Check sheet for the drawn part. Datum: minimum x, y, z corner. Units: mm. A direction names the side the tool comes from. Round coordinates to 2 decimals unless told otherwise and drop trailing zeros. Write each loop counter-clockwise with the first axis right and the second up, starting at its lowest first coordinate (ties: lowest second). Pieces come first, ordered by that corner, then holes. Notation, with made-up numbers: (-14, 46) - (-4, 46) arc R28 cw to (-4, 76) - close; hole circle Ø8 at (42, 63.25). An arc over 180 degrees is marked (long way). Write each question's results on one line, items separated by ' | '.
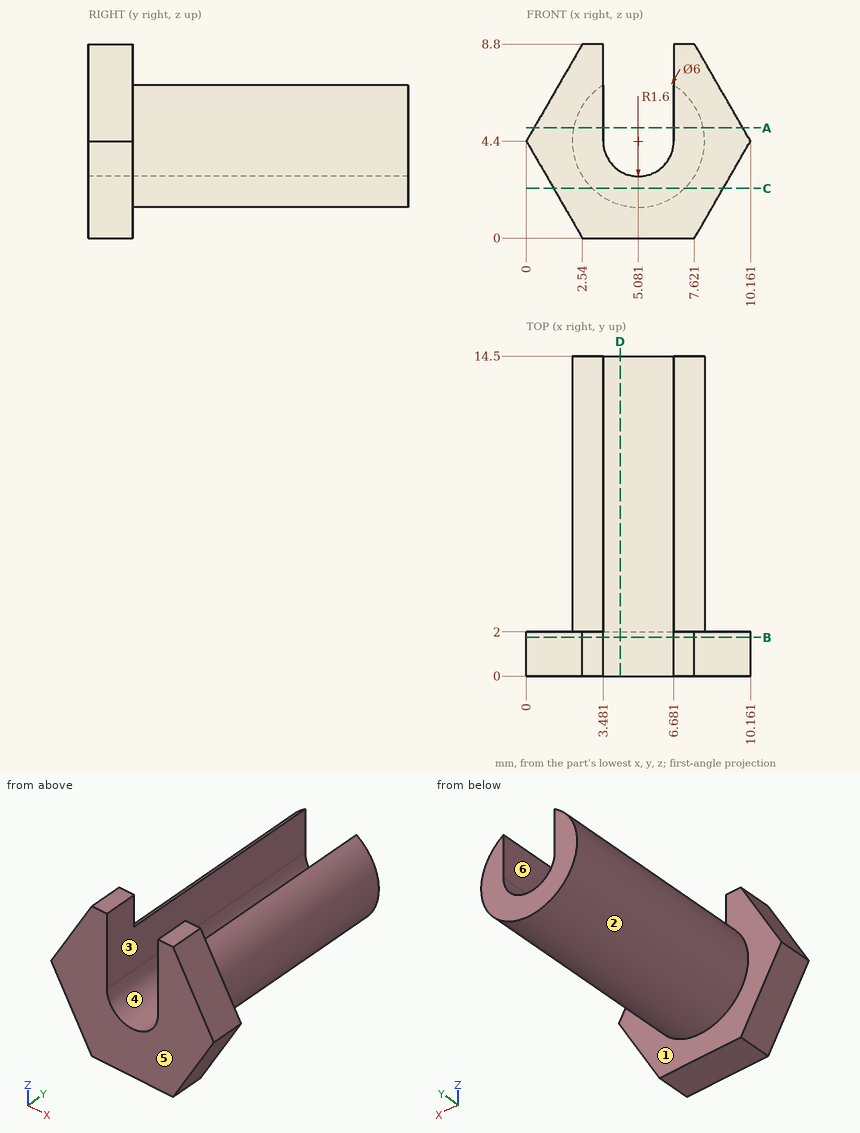
(1) Section check C-C (z = 2.25). Record the cut outline in (x, y).
Answer:
outline: (1.24, 0) - (8.92, 0) - (8.92, 2) - (7.17, 2) - (7.17, 14.5) - (2.99, 14.5) - (2.99, 2) - (1.24, 2) - close
(2) Set-up check for the marked faces 5 and 6: record each of +Z, -Z, +X, -X, +Y, -Y from which the full face is reachable in a straight line by a thin tool's end or side.
Answer:
face 5: +Z, -Z, +X, -X, -Y | face 6: +Z, +Y, -Y
(3) Mould release check, pull along X, two halves, no side actions. Record for the marked faces 1, 2, 3 and 4: released by +X, released by -X, zero draft, split by the parting line, or undercut.
Answer:
face 1: zero draft | face 2: split by the parting line | face 3: undercut | face 4: undercut
(4) Section check D-D (x = 4.25). Record the cut outline in (y, z), plus the area to 3 significant figures.
Answer:
outline: (0, 0) - (2, 0) - (2, 1.52) - (14.5, 1.52) - (14.5, 3.03) - (0, 3.03) - close | area: 25.0 mm2
(5) Section check B-B (y = 1.75). Record the cut outline in (x, z).
Answer:
outline: (0, 4.4) - (2.54, 0) - (7.62, 0) - (10.16, 4.4) - (7.62, 8.8) - (6.68, 8.8) - (6.68, 4.4) arc R1.6 cw to (3.48, 4.4) - (3.48, 8.8) - (2.54, 8.8) - close
(6) Section check A-A (z = 5). Record the cut outline in (x, y) (1 decimal).
Answer:
outline: (0.3, 0) - (3.5, 0) - (3.5, 14.5) - (2.1, 14.5) - (2.1, 2) - (0.3, 2) - close; (6.7, 0) - (9.8, 0) - (9.8, 2) - (8, 2) - (8, 14.5) - (6.7, 14.5) - close
(7) Thickness scan on L1, parallel to X at y = 11, z = 5.5; L2, parallel to X at y = 7, z = 5.75; L3, parallel to Y at x = 2, z = 7.5. Record the ranges inside material, lowest first.
Answer:
L1: 2.29 to 3.48, 6.68 to 7.87 | L2: 2.4 to 3.48, 6.68 to 7.76 | L3: 0 to 2
(8) Go/stop test with flat-tipped pins: pin 1 Ø6 at (x, y) = (1.5, 3) entering from -Z; pin 2 Ø1 at (x, y) = (6, 2) entering from +Z; pin 3 Ø2 at (y, z) = (1.5, 3) entering from -X; pin 4 Ø2 at (y, z) = (9, 6) entering from +X. Record where each tip stops, or that it passes through.
Answer:
pin 1: z = 0 | pin 2: z = 3.66 | pin 3: x = 0.23 | pin 4: x = 8.02
